from build123d import *
from build123d.topology import SkipClean

# Parameters (mm, degrees)
SKETCH1_R               = 73.66
SKETCH1_R_2             = 55.88
BOSS_EXTRUDE1_DEPTH     = 22.225
CUT_EXTRUDE1_REACH      = 108.515
SKETCH3_W               = 174.179431321
SKETCH3_H               = 95.128766337
F_1_4_CLEARANCE_HOLE1_D = 7.14248
SKETCH5_R               = 8.5
CUT_EXTRUDE2_DEPTH      = 56.1975
BOSS_EXTRUDE3_START     = 12.7
BOSS_EXTRUDE3_DEPTH     = 12.7
CUT_EXTRUDE3_DEPTH      = 31.925
FILLET1_R               = 5


with BuildPart() as part:
    # Sketch1 → Boss-Extrude1 (new body)
    with BuildSketch(Plane(origin=(0, 0, 0), x_dir=(1, 0, 0), z_dir=(0, 1, 0))):
        with Locations(Location((0, 0, 0), (0, 0, 270))):
            Circle(SKETCH1_R)
        with Locations(Location((0, 0, 0), (0, 0, 270))):
            Circle(SKETCH1_R_2, mode=Mode.SUBTRACT)
    extrude(amount=BOSS_EXTRUDE1_DEPTH)

    # Sketch3 → Cut-Extrude1 (cut, up to next)
    with BuildSketch(Plane(origin=(0, 22.225, 0), x_dir=(1, 0, 0), z_dir=(0, 1, 0)), mode=Mode.PRIVATE) as cut_extrude1_sk1:
        with Locations((-0.022555156, -42.801883168)):
            Rectangle(SKETCH3_W, SKETCH3_H)
    cut_extrude1_tool1 = extrude(cut_extrude1_sk1.sketch, amount=-CUT_EXTRUDE1_REACH, mode=Mode.PRIVATE) & part.part
    add(cut_extrude1_tool1.solids().sort_by_distance((-0.022555, 22.225, 42.801883))[0], mode=Mode.SUBTRACT)

    # 1/4 Clearance Hole1 (through all)
    with Locations(Plane(origin=(-64.591280655, 11.1125, -4.7625), x_dir=(1, 0, 0), z_dir=(0, 0, 1))):
        with Locations((0, 0), (129.18256131, 0)):
            Hole(F_1_4_CLEARANCE_HOLE1_D / 2)

    # Sketch5 → Cut-Extrude2 (cut)
    with BuildSketch(Plane(origin=(0, 0, -73.66), x_dir=(-1, 0, 0), z_dir=(0, 0, -1))):
        with Locations((-64.591280655, 11.1125)):
            Circle(SKETCH5_R)
        with Locations((64.591280655, 11.1125)):
            Circle(SKETCH5_R)
    extrude(amount=-CUT_EXTRUDE2_DEPTH, mode=Mode.SUBTRACT)

    # Sketch7 → Boss-Extrude3 (add)
    with SkipClean():  # the faces are left unmerged after this step: merging them gives an invalid solid
        with BuildSketch(Plane.XZ.offset(BOSS_EXTRUDE3_START)):
            with BuildLine():
                Line((73.505878634, -4.7625), (55.676682676, -4.7625))
                ThreePointArc((55.676682676, -4.7625), (0, -55.88), (-55.676682676, -4.7625))
                Line((-55.676682676, -4.7625), (-73.505878634, -4.7625))
                ThreePointArc((-73.505878634, -4.7625), (0, -73.66), (73.505878634, -4.7625))
            make_face()
        extrude(amount=-BOSS_EXTRUDE3_DEPTH)

    # Sketch9 → Cut-Extrude3 (cut)
    with SkipClean():  # the faces are left unmerged after this step: merging them gives an invalid solid
        with BuildSketch(Plane(origin=(0, 22.225, 0), x_dir=(1, 0, 0), z_dir=(0, 1, 0))):
            with BuildLine():
                Line((-50, 49.928304598), (-50, 31.094282433))
                ThreePointArc((-50, 31.094282433), (0, 58.88), (50, 31.094282433))
                Line((50, 31.094282433), (50, 49.928304598))
                ThreePointArc((50, 49.928304598), (0, 70.66), (-50, 49.928304598))
            make_face()
        extrude(amount=-CUT_EXTRUDE3_DEPTH, mode=Mode.SUBTRACT)

    # Fillet1
    fillet1_edges = [part.edges().sort_by_distance(p)[0] for p in [
        (-50, 6.2625, -31.094282433),
        (50, 6.2625, -31.094282433),
        (50, 6.2625, -49.928304598),
        (-50, 6.2625, -49.928304598),
    ]]
    fillet(fillet1_edges, radius=FILLET1_R)


solid = part.part
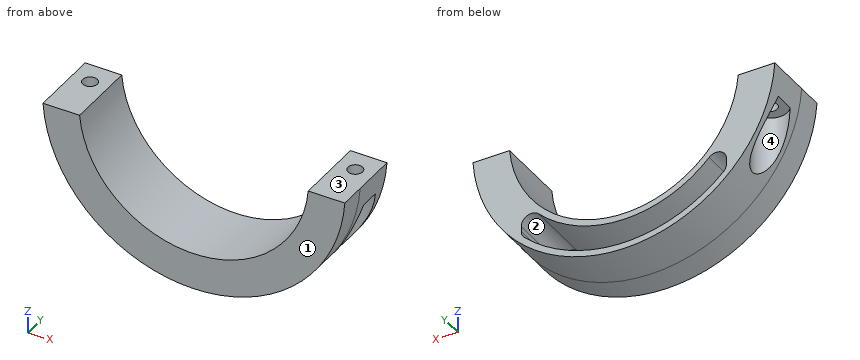
Geometry check sheet. Reference: the model listing, model coordinates, mm. Face numbers are marked on the shaded views. A direction names the side the tool comes from. Give positions to 0.01 mm unless a question says otherwise; leave off trailing zeros. Loops run counter-clockwise (first coordinate to the right, second up) from the corner with the lowest first, then second, coordinate; pieces in that order, holes last. Notation, with made-up numbers: (19.5, 42.25) -> (37.5, 42.25) arc R23 cw to (37.5, 81.25) -> close; hole circle Ø1 at (40.25, 67.25). An arc over 180 degrees is marked (long way). Answer in a Markdown table with one row per item. Add a question column.
1) Cross-section at A-A on y = -6.5. Record the boundary of the cut face in (x, z).
2) Cross-section at D-D on x = -39. Record the boundary of the cut face in (y, z) (3 decimals).
3) Gauge pin test, flat ends, axial feed: P1, Ø5, axis at x = 16, y = 7.5, coming from the -Z side; P2, Ø12, axis at y = 2, z = -17.5, coming from the -X side; P3, Ø8, axis at y = -1.5, z = -22, coming from the +X side. Record the tip position at first contact, or that the pin passes through.
4) Set-up check for the marked faces 1 and 2: record each of +Z, -Z, +X, -X, +Y, -Y from which the full face is reachable in a straight line by a thin tool's end or side.
5) Draft check along X on the marked faces 3 and 4. Enter one of: pulls with the +X half, pulls with the -X half, needs draft (parallel to the pull), parting line crosses it, or undercut.
6) Cross-section at C-C on x = 0. Record the boundary of the cut face in (y, z) (3 decimals), and give its area (3 significant figures).
7) Cross-section at B-B on z = -15. Record the boundary of the cut face in (x, y) (1 decimal).
8) Material ranges on probe 1 along X at (y, z) = (15, -41); probe 2 along X at (y, z) = (20.5, -47); probe 3 along X at (y, z) = (14.5, -17.5), recorded low to high. Write a range as from..to.
Outcome:
| question | item | result |
|---|---|---|
| 1 | outline | (-73.51, -4.76) arc R73.66 ccw to (73.51, -4.76) -> (55.68, -4.76) arc R55.88 cw to (-55.68, -4.76) -> close; hole (-50, -47.81) arc R5 ccw to (-48.43, -51.46) arc R70.66 ccw to (48.43, -51.46) arc R5 ccw to (50, -47.81) -> (50, -45.34) arc R5 ccw to (41.48, -41.79) arc R58.88 cw to (-41.48, -41.79) arc R5 ccw to (-50, -45.34) -> close |
| 2 | outline | (-12.7, -62.488) -> (22.225, -62.488) -> (22.225, -58.922) -> (-9.7, -58.922) -> (-9.7, -44.112) -> (22.225, -44.112) -> (22.225, -40.02) -> (-12.7, -40.02) -> close |
| 3 | P1 | stops at z = -72.41 |
| 3 | P2 | stops at x = -72.76 |
| 3 | P3 | stops at x = 71.43 |
| 4 | face 1 | +Z, -Z, +X, -X, -Y |
| 4 | face 2 | +Y |
| 5 | face 3 | needs draft |
| 5 | face 4 | undercut |
| 6 | outline | (-12.7, -73.66) -> (22.225, -73.66) -> (22.225, -70.66) -> (-9.7, -70.66) -> (-9.7, -58.88) -> (22.225, -58.88) -> (22.225, -55.88) -> (-12.7, -55.88) -> close |
| 6 | area | 245 mm^2 |
| 7 | outline | (-72.1, -12.7) -> (-53.8, -12.7) -> (-53.8, 22.2) -> (-72.1, 22.2) -> close; (53.8, -12.7) -> (72.1, -12.7) -> (72.1, 22.2) -> (53.8, 22.2) -> close; hole circle Ø7.1 at (-64.6, 11.1); hole circle Ø7.1 at (64.6, 11.1) |
| 8 | probe 1 | x = -57.03..-47.48, -42.52..-37.97, 37.97..42.52, 47.48..57.03 |
| 8 | probe 2 | x = -56.72..-50, -35.47..-30.23, 30.23..35.47, 50..56.72 |
| 8 | probe 3 | x = -56.8..-53.07, 53.07..56.8 |
